Autodesk Inventor part; units mm, degrees
ref_plane "YZ Plane" through (0, 0, 0) normal (1, 0, 0) x (0, 1, 0)
ref_plane "XZ Plane" through (0, 0, 0) normal (0, 1, 0) x (-1, 0, 0)
ref_plane "XY Plane" through (0, 0, 0) normal (0, 0, 1) x (1, 0, 0)
sketch "Sketch1" plane through (0, 0, 0) normal (0, 1, 0) x (-1, 0, 0)
  line L0 (0, 0) -> (88, 0)
  line L1 (88, 0) -> (88, -97)
  line L2 (88, -97) -> (0, -97)
  line L3 (0, -97) -> (0, 0)
  dimension "d0" = 97
  dimension "d1" = 88
extrude "Plate1" add sketch "Sketch1" along normal blind 1.5
sketch "Sketch2" plane through (-86.5, 0, 0) normal (-1, 0, 0) x (0, -1, 0)
  line L0 (0, -97) -> (0, 0)
  line L1 (0, 0) -> (-40, 0)
  line L2 (-40, 0) -> (-40, -97)
  line L3 (-40, -97) -> (0, -97)
edge flange "Flange1" height 40 angle 90 thickness 1.5 bend radius 1.5 thickness toward (-1, 0, 0) relief tear relief width 1.5 relief depth 0.75 corner gap 1.5 corner form 2 edges at (-88, 1.5, -48.5) (-44, 1.5, 0) (0, 1.5, -48.5) (-44, 1.5, -97) wall of the first edge with corners at (-86.5, 0, -97) (-86.5, 0, 0) (-86.5, 40, 0) (-86.5, 40, -97)
bend "Bend1"
corner "Corner1"
equation "\"d2\" = Thickness"
equation "\"d3\" = BendReliefWidth"
equation "\"d4\" = BendReliefDepth"
equation "\"d5\" = MinimumRemnant"
equation "\"d6\" = TransitionRadius"
equation "\"d9\" = BendRadius"
equation "\"d10\" = CornerReliefSize"
equation "\"d11\" = GapSize"
equation "\"d12\" = JacobiRadiusSize"
equation "\"BendRadius\" = Thickness"
equation "\"BendReliefWidth\" = Thickness"
equation "\"BendReliefDepth\" = 0.5 * Thickness"
equation "\"CornerReliefSize\" = 4 * Thickness"
equation "\"MinimumRemnant\" = 2 * Thickness"
equation "\"TransitionRadius\" = BendRadius"
equation "\"JacobiRadiusSize\" = BendRadius"
equation "\"GapSize\" = Thickness"
Build history of the part. All positions in model axes, mm. A direction names the side the tool comes from. Round coordinates to 2 decimals unless told otherwise and drop trailing zeros. Loops run counter-clockwise (first coordinate to the right, second up) from the corner with the lowest first, then second, coordinate; pieces in that order, holes last. Notation, with made-up numbers: (15.25, 5) -> (50.25, 5) arc R28 ccw to (50.25, 37) -> close; hole circle Ø8 at (87, -30). An arc over 180 degrees is marked (long way). Use CSV: the item, a comma, the result in double quotes. Start each with the question number.
Q1. Saw through at B-B on z = -60. Give the cut face in (x, y).
Q2. Saw through at C-C on x = -17. Give the cut face in (y, z).
Q3. Which spindle directions (+Z, -Z, +X, -X, +Y, -Y) get a long thin tool onto all of the face, cutting with end or side? Do faces 5 (the face through (-86.5, 1.5, -3)), 6 (the face through (-86.5, 21, -48)), 7 (the face through (-85, 1.5, -95.5)). Say none if no direction does.
Q4. Saw through at A-A on y = 33.5. Give the cut face in (x, z), and give its area (3 significant figures).
Q5. Flat gauge pins, fed straight in: pin 1 Ø2.5 at (x, y) = (-86, 1) entering from -Z; pin 2 Ø0.5 at (x, z) = (-85.5, -96.5) entering from -Y; pin 3 Ø1 at (x, z) = (-46, -52) entering from +Y. Where does each tip first touch, or does it go through?
Q6. Mould opens along Z. For faces 1 (the face through (-45, 21, -95.5)), 2 (the face through (-88, 22, -48)), 3 (the face through (-43, 1.5, -48)), 4 (the face through (-1.5, 1.5, -94)) say: +Z half, -Z half, draft (parallel to the pull), parting line (faces both ways), or undercut.
Q7. Drill centre lines: L1, parallel to X at y = 6, z = -68.5; L2, parallel to Z at x = -15.5, y = 21.5; L3, parallel to Y at x = -16, z = -14.5. Where is each one in solid material? Low to high.
Solutions:
1,outline,"(-88, 3) arc R3 ccw to (-85, 0) -> (-3, 0) arc R3 ccw to (0, 3) -> (0, 40) -> (-1.5, 40) -> (-1.5, 3) arc R1.5 cw to (-3, 1.5) -> (-85, 1.5) arc R1.5 cw to (-86.5, 3) -> (-86.5, 40) -> (-88, 40) -> close"
2,outline,"(0, -94) arc R3 ccw to (3, -97) -> (40, -97) -> (40, -95.5) -> (3, -95.5) arc R1.5 cw to (1.5, -94) -> (1.5, -3) arc R1.5 cw to (3, -1.5) -> (40, -1.5) -> (40, 0) -> (3, 0) arc R3 ccw to (0, -3) -> close"
3,face 5,"+Z, -X, -Y"
3,face 6,"+Z, -Z, +Y"
3,face 7,"-Z, -X, -Y"
4,outline,"(-88, -94.44) -> (-86.5, -94.44) -> (-86.5, -2.56) -> (-88, -2.56) -> close; (-85.44, -97) -> (-2.56, -97) -> (-2.56, -95.5) -> (-85.44, -95.5) -> close; (-85.44, -1.5) -> (-2.56, -1.5) -> (-2.56, 0) -> (-85.44, 0) -> close; (-1.5, -94.44) -> (0, -94.44) -> (0, -2.56) -> (-1.5, -2.56) -> close"
4,area,"524 mm^2"
5,pin 1,"stops at z = -96.73"
5,pin 2,"stops at y = 3"
5,pin 3,"stops at y = 1.5"
6,face 1,"undercut"
6,face 2,"draft"
6,face 3,"undercut"
6,face 4,"-Z half"
7,L1,"x = -88 to -86.5, -1.5 to 0"
7,L2,"z = -97 to -95.5, -1.5 to 0"
7,L3,"y = 0 to 1.5"
